```python
from build123d import *

# Parameters (mm, degrees)
F0_W     = 20
F0_H     = 3.05
F0_W_2   = 3.05
F0_H_2   = 20
F1_DEPTH = 3


with BuildPart() as f1:
    # F0 (on Right) → F1 (new body)
    with BuildSketch(Plane.YZ):
        Polygon((10, -35), (21, -35), (21, -10), (21, 10), (21, 35), (10, 35), (-10, 35), (-21, 35), (-21, -35), (-10, -35), align=None)
        with Locations((0, -36.525)):
            Rectangle(F0_W, F0_H)
        with Locations((22.525, 0)):
            Rectangle(F0_W_2, F0_H_2)
        with Locations((0, 36.525)):
            Rectangle(F0_W, F0_H)
    extrude(amount=F1_DEPTH)


solid = f1.part
```
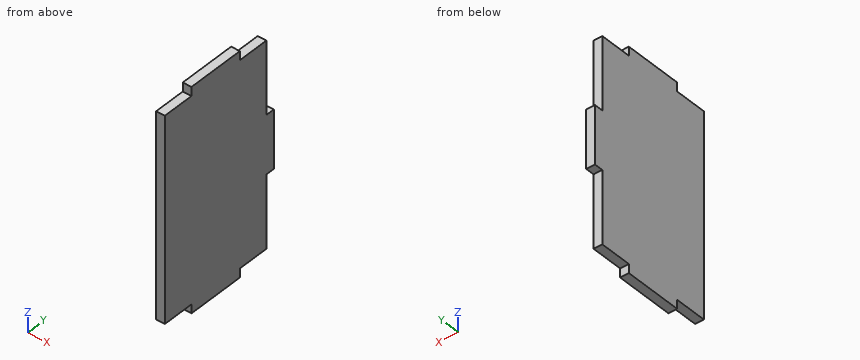
Geometry: final body of the model. Coordinates: model frame, mm. Give positions to 0.01 mm unless a question says otherwise; leave off trailing zeros. Loops run counter-clockwise (first coordinate to the right, second up) from the corner with the lowest first, then second, coordinate; pieces in that order, holes last. Notation, with made-up numbers: (60, -11) - (98, -11) arc R27 ccw to (98, 18) - close; hole circle Ø2 at (-28, 87). An arc over 180 degrees is marked (long way). Answer as CSV lines item,"result". Start each with the question number.
(1) Pin query (flat end, axial travel): P1, Ø1, axis at x = 1, y = -12, coming from the +Z side; P2, Ø0.9, axis at x = 1.5, z = -37, coming from the -Y side; P3, Ø1.5, axis at x = 1.5, z = -36.5, coming from the +Y side. Return the tip coordinate at first contact, or that it passes through.
(2) Ray query, line 1 along Z through (x, y) = (0.5, -12.5); line 2 along Y through (x, z) = (2.05, 28); line 3 along Y through (x, z) = (1.95, 35.5). Return the intervals inside material, ascending. Write a range as [from, to].
(3) Section query A-A (x = 1.2). Output: boundary loops of the cut face in (y, z), and give its area (3 significant figures).
(4) Section query B-B (z = -22). Output: boundary loops of the cut face in (x, y).
(5) Section query C-C (y = -12.5). Output: boundary loops of the cut face in (x, z).
Worked answers:
1,P1,"stops at z = 35"
1,P2,"stops at y = -10"
1,P3,"stops at y = 10"
2,line 1,"z = [-35, 35]"
2,line 2,"y = [-21, 21]"
2,line 3,"y = [-10, 10]"
3,outline,"(-21, -35) - (-10, -35) - (-10, -38.05) - (10, -38.05) - (10, -35) - (21, -35) - (21, -10) - (24.05, -10) - (24.05, 10) - (21, 10) - (21, 35) - (10, 35) - (10, 38.05) - (-10, 38.05) - (-10, 35) - (-21, 35) - close"
3,area,"3,120 mm^2"
4,outline,"(0, -21) - (3, -21) - (3, 21) - (0, 21) - close"
5,outline,"(0, -35) - (3, -35) - (3, 35) - (0, 35) - close"
